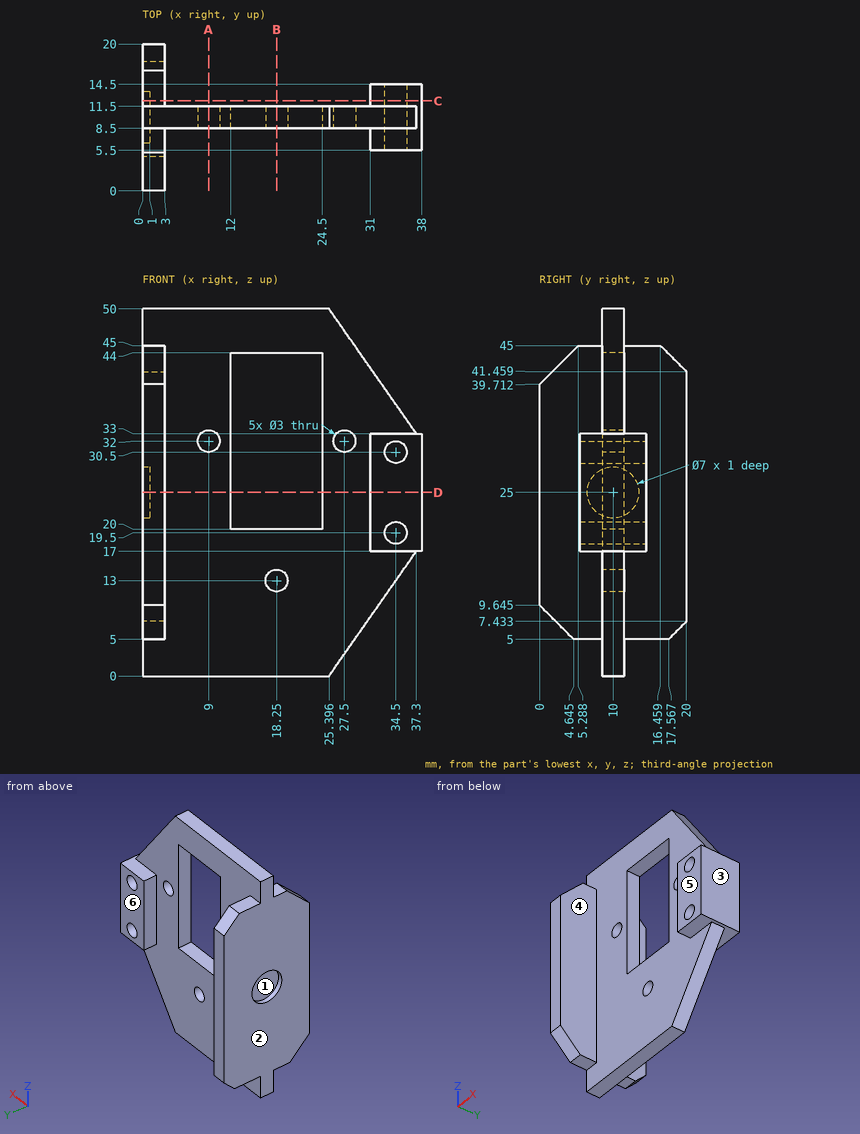
Verification items for this drawing (mm, ordinates from the low corner). A direction names the side the tool comes from. Round coordinates to 2 decimals unless told otherwise and drop trailing zeros. Order: outer loops, then holes, each group sorted by start corner. A loop starts at its lowest first (then second) coordinate and runs counter-clockwise, first axis right, second up. Notation, with made-up numbers: (23.25, -38) - (44.25, -38) arc R33 cw to (44.25, -9) - close; hole circle Ø7 at (25, 66). An arc over 180 degrees is marked (long way). Use CSV: the item, a comma, the result in double quotes. Start each with the question number.
1) Section check C-C, the plane y = 12.25. Record the cut outline in (x, z).
2) Go/stop test with flat-tipped pins: P1, Ø1.8, axis at x = 9, z = 32, coming from the +Y side; P2, Ø5.5, axis at x = 33.5, z = 21.5, coming from the -Y side; P3, Ø1.5, axis at x = 13.5, z = 13.5, coming from the -Y side; P4, Ø5.5, axis at y = 10, z = 25, coming from the -X side. Record where each tip stops, or that it passes through.
3) Section check B-B, the plane x = 18.25. Record the cut outline in (y, z), plus the area to 3 significant figures.
4) Access from +Z, -Z, +X, -X, +Y, -Y to the whole of each face (thin tool, end or side, straight path). Record for the marked faces 3, 4, 5 and 6.
5) Mould release check, pull along Z, two halves, no side actions. Record for the marked faces 1 and 2: +Z half, -Z half, draft (parallel to the pull), parting line (faces both ways), or undercut.
6) Thickness scan on L1, parallel to Z at x = 18.25, y = 9.3; L2, parallel to X at y = 9.5, z = 19.5; L3, parallel to X at y = 3.75, z = 16. Record the ranges inside material, lowest first.
7) Section check A-A, the plane x = 9. Record the cut outline in (y, z).
8) Section check D-D, the plane z = 25. Record the cut outline in (x, y).
Answers:
1,outline,"(0, 5) - (3, 5) - (3, 45) - (0, 45) - (0, 27.68) - (1, 27.68) - (1, 22.32) - (0, 22.32) - close; (31, 17) - (38, 17) - (38, 33) - (31, 33) - close; hole circle Ø3 at (34.5, 19.5); hole circle Ø3 at (34.5, 30.5)"
2,P1,"passes through"
2,P2,"stops at y = 5.5"
2,P3,"stops at y = 8.5"
2,P4,"stops at x = 1"
3,outline,"(8.5, 0) - (11.5, 0) - (11.5, 11.5) - (8.5, 11.5) - close; (8.5, 14.5) - (11.5, 14.5) - (11.5, 20) - (8.5, 20) - close; (8.5, 44) - (11.5, 44) - (11.5, 50) - (8.5, 50) - close"
3,area,"69.0 mm²"
4,face 3,"+Z, -Z, +X, +Y, -Y"
4,face 4,"+Z, -Z, -Y"
4,face 5,"+Z, -Z, +X, -Y"
4,face 6,"+Z, -Z, +X, +Y"
5,face 1,"undercut"
5,face 2,"draft"
6,L1,"z = 0 to 11.5, 14.5 to 20, 44 to 50"
6,L2,"x = 0 to 33, 36 to 38"
6,L3,"x = 0 to 3"
7,outline,"(8.5, 0) - (11.5, 0) - (11.5, 30.5) - (8.5, 30.5) - close; (8.5, 33.5) - (11.5, 33.5) - (11.5, 50) - (8.5, 50) - close"
8,outline,"(0, 0) - (3, 0) - (3, 8.5) - (12, 8.5) - (12, 11.5) - (3, 11.5) - (3, 20) - (0, 20) - (0, 13.5) - (1, 13.5) - (1, 6.5) - (0, 6.5) - close; (24.5, 8.5) - (31, 8.5) - (31, 5.5) - (38, 5.5) - (38, 14.5) - (31, 14.5) - (31, 11.5) - (24.5, 11.5) - close"
